Source: CAD feature listing. Evaluate the final solid. Frame: model axes, mm. A direction names the side the tool comes from. Give positions to 0.01 mm unless a question says otherwise; leave off trailing zeros. Loops run counter-clockwise (first coordinate to the right, second up) from the corner with the lowest first, then second, coordinate; pieces in that order, holes last. Notation, with made-up numbers: (4, 82.25) - (16, 82.25) arc R24 ccw to (16, 118.25) - close; hole circle Ø11 at (26.5, -37). An arc over 180 degrees is marked (long way). Write each question's results on one line, items separated by ' | '. Start each with the question number.
(1) Cut plane B-B on z = -7.5. Return the cut outline in (x, y) (3 decimals), then the cut area to 3 significant figures.
(2) Material intervals for line 1 along Z through (x, y) = (3.75, 2.1); line 2 along Z through (x, y) = (-3.75, 1.6); line 3 along X through (y, z) = (1.8, -35), sorted ascending. Write a range as [from, to].
(3) Cut plane A-A on z = -35. Return the cut outline in (x, y) (3 decimals), then the cut area to 3 significant figures.
(4) Pull-direction query (X, two-part tool) for faces 1 (the flat face through (-2.5, 1, 47)), 2 (the cylindrical face through (-2.113, 1.895, -34.253)), 3 (the flat face through (0, 0, 1)), 4 (the flat face through (2.5, 1, 47)); classes: pulls with the +X half, pulls with the -X half, needs draft (parallel to the pull), parting line crosses it, or undercut.
(5) Reachability of faces 5 (the flat face through (0, 3, -46)), 6 (the flat face through (-6, 3, 1)), 7 (the flat face through (2.5, 1, -48)) from +Z, -Z, +X, -X, +Y, -Y: full face, straight path, thin tool, end or side. Return the list, or none.
(6) Contact query for flat-ended pins moving along their axis: pin 1 (1 mm diameter, centred on x = 0.5, z = 22, fed in from +Y); pin 2 (5.5 mm diameter, centred on x = -0.5, z = 46, fed in from +Y); pin 3 (2 mm diameter, centred on x = 0, z = -49.5, fed in from +Y); pin 4 (2.5 mm diameter, centred on y = 1.5, z = -49.5, fed in from -X). Output: stop coordinate, or through.
(7) Cut plane C-C on z = -49.5. Return the cut outline in (x, y).
from build123d import *

# Parameters (mm, degrees)
SKETCH1_W               = 5
SKETCH1_H               = 85
BOSS_EXTRUDE1_DEPTH     = 3
BOSS_EXTRUDE2_DEPTH     = 42.5
BOSS_EXTRUDE3_START     = 42.5
BOSS_EXTRUDE3_DEPTH     = 42.5
SKETCH8_W               = 5
SKETCH8_H               = 10
BOSS_EXTRUDE4_DEPTH     = 3
SKETCH6_R               = 1.8
CUT_EXTRUDE1_DEPTH      = 53.645037753
SKETCH9_W               = 15
SKETCH9_H               = 85
BOSS_EXTRUDE5_DEPTH     = 3
FILLET1_R               = 1
CUT_EXTRUDE2_DEPTH      = 54.117793629
CUT_EXTRUDE2_DEPTH_BACK = 54.117793629
SKETCH10_R              = 1.8


with BuildPart() as part:
    # Sketch1 → Boss-Extrude1 (new body)
    with BuildSketch(Plane(origin=(0, 0, 0), x_dir=(1, 0, 0), z_dir=(0, 1, 0))):
        Rectangle(SKETCH1_W, SKETCH1_H)
    extrude(amount=BOSS_EXTRUDE1_DEPTH)

    # Sketch3 → Boss-Extrude2 (add)
    with BuildSketch(Plane.XY):
        with BuildLine():
            Line((-2.5, 3), (-2.5, 5.102989898))
            ThreePointArc((-2.5, 5.102989898), (0, 5.05), (2.5, 5.102989898))
            Line((2.5, 5.102989898), (2.5, 3))
            Line((2.5, 3), (2.5, 0))
            Line((2.5, 0), (-2.5, 0))
            Line((-2.5, 0), (-2.5, 3))
        make_face()
    extrude(amount=BOSS_EXTRUDE2_DEPTH)

    # Sketch7 → Boss-Extrude3 (add)
    with BuildSketch(Plane(origin=(0, 0, 0), x_dir=(-1, 0, 0), z_dir=(0, 0, -1)).offset(BOSS_EXTRUDE3_START)):
        with BuildLine():
            Line((-2.5, 5.102989898), (-2.5, 3))
            Line((-2.5, 3), (2.5, 3))
            Line((2.5, 3), (2.5, 5.102989898))
            ThreePointArc((2.5, 5.102989898), (0, 5.05), (-2.5, 5.102989898))
        make_face()
    extrude(amount=-BOSS_EXTRUDE3_DEPTH)

    # Sketch8 → Boss-Extrude4 (add)
    with BuildSketch(Plane.XZ):
        with Locations((0, 47.5)):
            Rectangle(SKETCH8_W, SKETCH8_H)
        with Locations((0, -47.5)):
            Rectangle(SKETCH8_W, SKETCH8_H)
    extrude(amount=-BOSS_EXTRUDE4_DEPTH)

    # Sketch6 → Cut-Extrude1 (cut, through all)
    with BuildSketch(Plane(origin=(0, 3, 0), x_dir=(1, 0, 0), z_dir=(0, 1, 0))):
        with Locations(Location((0, -49.5, 0), (0, 0, 270))):
            Circle(SKETCH6_R)
        with Locations(Location((0, 49.5, 0), (0, 0, 90))):
            Circle(SKETCH6_R)
    extrude(amount=-CUT_EXTRUDE1_DEPTH, mode=Mode.SUBTRACT)

    # Sketch9 → Boss-Extrude5 (add)
    with BuildSketch(Plane.XZ):
        Rectangle(SKETCH9_W, SKETCH9_H)
    extrude(amount=-BOSS_EXTRUDE5_DEPTH)

    # Fillet1
    # the kernel refuses this fillet: 1 mm, written as the material it adds along each edge
    with BuildSketch(Plane(origin=(2.5, 3, -42.5), x_dir=(0, 1, 0), z_dir=(0, 0, 1)), Plane(origin=(-2.5, 3, 42.5), x_dir=(0, 1, 0), z_dir=(0, 0, -1))) as fillet1_piece_1:
        with BuildLine():
            CenterArc((FILLET1_R, -FILLET1_R), FILLET1_R, 90, 90)
            Line((0, -FILLET1_R), (0, 0))
            Line((0, 0), (FILLET1_R, 0))
        make_face()
    extrude(amount=85)
    # the kernel refuses this fillet: 1 mm, written as the material it takes off along each edge
    with BuildSketch(Plane(origin=(-2.5, 5.102989898, 45.085592418), x_dir=(0, -1, 0), z_dir=(0, 0, -1))) as fillet1_2_piece_1:
        with BuildLine():
            CenterArc((1.034236967, -1), FILLET1_R, 90, 91.432543738)
            ThreePointArc((0.034549516, -1.025), (0.019501965, -0.512424928), (0, 0))
            Line((0, 0), (1.034236967, 0))
        make_face()
    extrude(amount=90.171184836, mode=Mode.SUBTRACT)
    with BuildSketch(Plane(origin=(2.5, 5.102989898, 45.085592418), x_dir=(0, -1, 0), z_dir=(0, 0, -1))) as fillet1_2_piece_2:
        with BuildLine():
            CenterArc((1.034236967, 1), FILLET1_R, 178.567456262, 91.432543738)
            ThreePointArc((0.034549516, 1.025), (0.019501965, 0.512424928), (0, 0))
            Line((0, 0), (1.034236967, 0))
        make_face()
    extrude(amount=90.171184836, mode=Mode.SUBTRACT)

    # Sketch10 → Cut-Extrude2 (cut, two sides: drawn at the far end of the back side and taken through both)
    with BuildSketch(Plane(origin=(0, 3, 0), x_dir=(1, 0, 0), z_dir=(0, 1, 0)).offset(-CUT_EXTRUDE2_DEPTH_BACK)):
        with Locations(Location((-3.75, -35, 0), (0, 0, 270))):
            Circle(SKETCH10_R)
        with Locations(Location((3.75, -29, 0), (0, 0, 270))):
            Circle(SKETCH10_R)
        with Locations(Location((3.75, 29, 0), (0, 0, 262.016443854))):
            Circle(SKETCH10_R)
        with Locations(Location((-3.75, 35, 0), (0, 0, 277.983556156))):
            Circle(SKETCH10_R)
    extrude(amount=CUT_EXTRUDE2_DEPTH + CUT_EXTRUDE2_DEPTH_BACK, mode=Mode.SUBTRACT)


solid = part.part
Ans:
1) outline: (-7.5, 0) - (7.5, 0) - (7.5, 3) - (3.5, 3) arc R1 cw to (2.5, 4) - (2.5, 4.069) arc R1 ccw to (1.475, 5.068) arc R59 cw to (-1.475, 5.068) arc R1 ccw to (-2.5, 4.069) - (-2.5, 4) arc R1 cw to (-3.5, 3) - (-7.5, 3) - close | area: 55.3 mm^2
2) line 1: [-42.5, -30.8], [-27.2, 27.2], [30.8, 42.5] | line 2: [-42.5, -36.8], [-33.2, 33.2], [36.8, 42.5] | line 3: [-7.5, -5.55], [-1.95, 7.5]
3) outline: (-7.5, 0) - (-5.55, 0) - (-5.55, 3) - (-7.5, 3) - close; (-1.95, 0) - (7.5, 0) - (7.5, 3) - (3.5, 3) arc R1 cw to (2.5, 4) - (2.5, 4.069) arc R1 ccw to (1.475, 5.068) arc R59 cw to (-1.475, 5.068) arc R1 ccw to (-1.95, 4.962) - close | area: 43.4 mm^2
4) face 1: pulls with the -X half | face 2: undercut | face 3: needs draft | face 4: pulls with the +X half
5) face 5: -Z, +X, -X, +Y | face 6: +Z, -Z, -X, +Y | face 7: -Z, +X, +Y, -Y
6) pin 1: y = 5.06 | pin 2: y = 3 | pin 3: through | pin 4: x = -2.5
7) outline: (-2.5, 0) - (-1.8, 0) - (-1.8, 3) - (-2.5, 3) - close; (1.8, 0) - (2.5, 0) - (2.5, 3) - (1.8, 3) - close
